Study the drawing (mm; zero at the part's minimum x, y, z) and answer. Give positions to 0.01 mm unless a question says otherwise; leave off trailing zeros. Write each loop counter-clockwise with the first axis right and the second up, starting at its lowest first coordinate (ties: lowest second). Pieces come first, ordered by that corner, then holes.
1) Find section B-B (z = 21.5). Determine the outline of the cut face in (x, y), plus the area to 3 significant figures.
2) Determine the mould class of the marked faces 1 and 2 for opening direction X: pulls with the +X half, pulls with the -X half, needs draft (parallel to the pull), parting line crosses it, or undercut.
3) Find section A-A (x = 43). Determine the outline of the cut face in (y, z).
4) Straight lines are drawn through the part: probe 1 along Z at (x, y) = (62, 1.05); probe 2 along X at (y, z) = (2.7, 10.5); probe 3 along X at (y, z) = (4.8, 53). For each, find the intervals that lie inside material, in ascending order.
5) Given pin 1 Ø2 at (y, z) = (5, 37) entering from -X, flat-ended and moving along its own axis, determine where the tip first touches the part or whether it passes through.
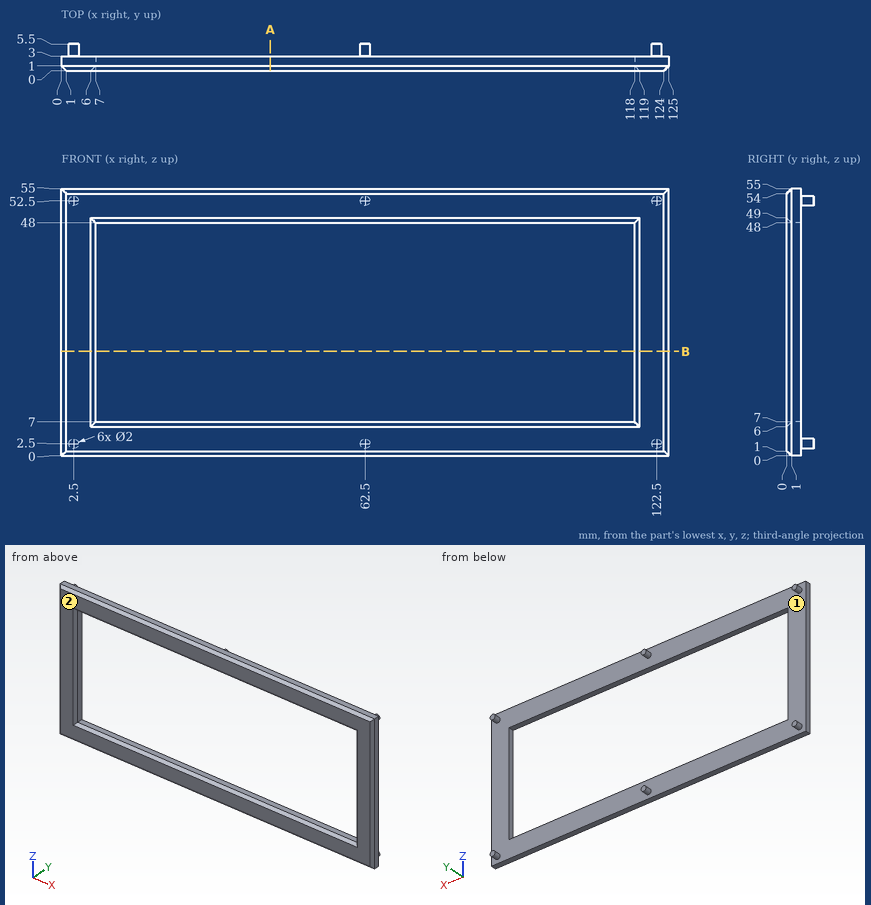
Results:
1. outline: (0, 1) - (1, 0) - (6, 0) - (7, 1) - (7, 3) - (0, 3) - close; (118, 1) - (119, 0) - (124, 0) - (125, 1) - (125, 3) - (118, 3) - close
1. area: 40.0 mm2
2. face 1: undercut
2. face 2: needs draft
3. outline: (0, 1) - (1, 0) - (3, 0) - (3, 7) - (1, 7) - (0, 6) - close; (0, 49) - (1, 48) - (3, 48) - (3, 55) - (1, 55) - (0, 54) - close
4. probe 1: z = 0 to 7, 48 to 55
4. probe 2: x = 0 to 7, 118 to 125
4. probe 3: x = 1.63 to 3.37, 61.63 to 63.37, 121.63 to 123.37
5. pin 1: passes through
